from build123d import *

# Parameters (mm, degrees)
SKETCH_1_W          = 44.75
SKETCH_1_H          = 50
EXTRUDE_1_DEPTH     = 30
SHELL_1_T           = 5
FILLET_1_R          = 5
SKETCH_2_R          = 0.75
CUT_EXTRUDE_1_DEPTH = 70.264438928
SKETCH_3_R          = 5
CUT_EXTRUDE_2_DEPTH = 70.264438928
EXTRUDE_2_DEPTH     = 30
CUT_EXTRUDE_3_DEPTH = 20
SKETCH_7_R          = 2.1
CUT_EXTRUDE_4_DEPTH = 159.731347329
SKETCH_8_W          = 18
SKETCH_8_H          = 45
CUT_EXTRUDE_5_DEPTH = 10
SKETCH_9_W          = 18
SKETCH_9_H          = 45
CUT_EXTRUDE_6_DEPTH = 10
FILLET_2_R          = 3


with BuildPart() as part:
    # 草图1 → 凸台-拉伸1 (new body)
    with BuildSketch(Plane.XY):
        Rectangle(SKETCH_1_W, SKETCH_1_H)
    extrude(amount=EXTRUDE_1_DEPTH)

    # 抽壳1
    shell_1_openings = [part.faces().sort_by_distance(p)[0] for p in [
        (0, -25, 15),
        (0, 0, 0),
        (0, 0, 30),
    ]]
    offset(amount=SHELL_1_T, openings=shell_1_openings, kind=Kind.INTERSECTION)

    # 圆角1
    # the kernel refuses this fillet: 5 mm, written as the material it takes off along each edge
    with BuildSketch(Plane(origin=(-27.375, 30, -12.5), x_dir=(1, 0, 0), z_dir=(0, 0, 1)), Plane(origin=(-27.375, -25, 42.5), x_dir=(1, 0, 0), z_dir=(0, 0, -1)), Plane(origin=(27.375, -25, -12.5), x_dir=(-1, 0, 0), z_dir=(0, 0, 1)), Plane(origin=(27.375, 30, 42.5), x_dir=(-1, 0, 0), z_dir=(0, 0, -1))) as fillet_1_piece_1:
        with BuildLine():
            CenterArc((FILLET_1_R, -FILLET_1_R), FILLET_1_R, 90, 90)
            Line((0, -FILLET_1_R), (0, 0))
            Line((0, 0), (FILLET_1_R, 0))
        make_face()
    extrude(amount=55, mode=Mode.SUBTRACT)
    with BuildSketch(Plane(origin=(-27.375, -37.5, 30), x_dir=(1, 0, 0), z_dir=(0, 1, 0)), Plane(origin=(27.375, 42.5, 30), x_dir=(-1, 0, 0), z_dir=(0, -1, 0))) as fillet_1_piece_2:
        with BuildLine():
            CenterArc((FILLET_1_R, FILLET_1_R), FILLET_1_R, 180, 90)
            Line((0, FILLET_1_R), (0, 0))
            Line((0, 0), (FILLET_1_R, 0))
        make_face()
    extrude(amount=80, mode=Mode.SUBTRACT)
    with BuildSketch(Plane(origin=(-27.375, -37.5, 0), x_dir=(1, 0, 0), z_dir=(0, 1, 0)), Plane(origin=(27.375, 42.5, 0), x_dir=(-1, 0, 0), z_dir=(0, -1, 0))) as fillet_1_piece_3:
        with BuildLine():
            CenterArc((FILLET_1_R, -FILLET_1_R), FILLET_1_R, 90, 90)
            Line((0, -FILLET_1_R), (0, 0))
            Line((0, 0), (FILLET_1_R, 0))
        make_face()
    extrude(amount=80, mode=Mode.SUBTRACT)

    # 草图2 → 切除-拉伸1 (cut, through all)
    with BuildSketch(Plane.ZY.offset(27.375)):
        with Locations(Location((15, 7, 0), (0, 0, 270))):
            Circle(SKETCH_2_R)
        with Locations(Location((12, 7, 0), (0, 0, 270))):
            Circle(SKETCH_2_R)
        with Locations(Location((18, 7, 0), (0, 0, 270))):
            Circle(SKETCH_2_R)
        with Locations(Location((8, -3, 0), (0, 0, 90))):
            Circle(SKETCH_2_R)
        with Locations(Location((8, 0, 0), (0, 0, 90))):
            Circle(SKETCH_2_R)
        with Locations(Location((8, 3, 0), (0, 0, 90))):
            Circle(SKETCH_2_R)
        with Locations(Location((12, -7, 0), (0, 0, 90))):
            Circle(SKETCH_2_R)
        with Locations(Location((15, -7, 0), (0, 0, 90))):
            Circle(SKETCH_2_R)
        with Locations(Location((18, -7, 0), (0, 0, 90))):
            Circle(SKETCH_2_R)
        with Locations(Location((22, -3, 0), (0, 0, 270))):
            Circle(SKETCH_2_R)
        with Locations(Location((22, 0, 0), (0, 0, 270))):
            Circle(SKETCH_2_R)
        with Locations(Location((22, 3, 0), (0, 0, 270))):
            Circle(SKETCH_2_R)
    extrude(amount=-CUT_EXTRUDE_1_DEPTH, mode=Mode.SUBTRACT)

    # 草图3 → 切除-拉伸2 (cut, through all)
    with BuildSketch(Plane(origin=(27.375, 0, 0), x_dir=(0, 0, -1), z_dir=(1, 0, 0))):
        with Locations(Location((-15, 0, 0), (0, 0, 90))):
            Circle(SKETCH_3_R)
    extrude(amount=-CUT_EXTRUDE_2_DEPTH, mode=Mode.SUBTRACT)

    # 草图4 → 凸台-拉伸2 (add)
    with BuildSketch(Plane.XY.offset(30)):
        Polygon((0, 30), (-15, 30), (-15, 150), (15, 150), (15, 30), align=None)
    extrude(amount=-EXTRUDE_2_DEPTH)

    # 草图6 → 切除-拉伸3 (cut)
    with BuildSketch(Plane.XY.offset(30)):
        Polygon((-15, 99), (15, 99), (15, 141), (5, 141), (5, 150), (-15, 150), (-15, 141), align=None)
    extrude(amount=-CUT_EXTRUDE_3_DEPTH, mode=Mode.SUBTRACT)

    # 草图7 → 切除-拉伸4 (cut, through all)
    with BuildSketch(Plane(origin=(15, 0, 0), x_dir=(0, 0, -1), z_dir=(1, 0, 0))):
        with Locations((-24.925, 144.75)):
            Circle(SKETCH_7_R)
        with Locations((-15.075, 144.75)):
            Circle(SKETCH_7_R)
        with Locations(Location((-15.075, 95.25, 0), (0, 0, 180))):
            Circle(SKETCH_7_R)
        with Locations(Location((-24.925, 95.25, 0), (0, 0, 180))):
            Circle(SKETCH_7_R)
    extrude(amount=-CUT_EXTRUDE_4_DEPTH, mode=Mode.SUBTRACT)

    # 草图8 → 切除-拉伸5 (cut)
    with BuildSketch(Plane.XY.offset(30)):
        with Locations((0, 64.5)):
            Rectangle(SKETCH_8_W, SKETCH_8_H)
    extrude(amount=-CUT_EXTRUDE_5_DEPTH, mode=Mode.SUBTRACT)

    # 草图9 → 切除-拉伸6 (cut)
    with BuildSketch(Plane(origin=(0, 0, 0), x_dir=(-1, 0, 0), z_dir=(0, 0, -1))):
        with Locations((0, 65)):
            Rectangle(SKETCH_9_W, SKETCH_9_H)
    extrude(amount=-CUT_EXTRUDE_6_DEPTH, mode=Mode.SUBTRACT)

    # 圆角2
    fillet_2_edges = [part.edges().sort_by_distance(p)[0] for p in [
        (-15, 90, 0),
        (15, 90, 0),
        (15, 64.5, 30),
        (-15, 64.5, 30),
    ]]
    fillet(fillet_2_edges, radius=FILLET_2_R)


solid = part.part
Geometry check sheet. Reference: the model listing, model coordinates, mm. A direction names the side the tool comes from. Give positions to 0.01 mm unless a question says otherwise; leave off trailing zeros. Loops run counter-clockwise (first coordinate to the right, second up) from the corner with the lowest first, then second, coordinate; pieces in that order, holes last. Notation, with made-up numbers: (64.25, -27.5) -> (97.25, -27.5) arc R4 ccw to (97.25, -21.5) -> close; hole circle Ø4 at (36.5, 75). An arc over 180 degrees is marked (long way). Answer in a Markdown table with one row per item. Add a question column.
1) Cross-section at C-C on y = -10.5. Record the boundary of the cut face in (x, z) (3 decimals).
2) Cross-section at D-D on y = 103. Record the boundary of the cut face in (x, z), and give its area (3 significant figures).
3) Cross-section at B-B on x = 6.5. Record the boundary of the cut face in (y, z) (3 decimals), and give its area (3 significant figures).
4) Set-up check for faces 4 (the face through (5, 145, 20)), 5 (the face through (0, 87.5, 5)), 6 (the face through (14.1, 89.16, 0.86)), 7 (the face through (-22.375, -6, 15)): record each of +Z, -Z, +X, -X, +Y, -Y from which the full face is reachable in a straight line by a thin tool's end or side.
5) Gauge pin test, flat ends, axial feed: P1, Ø2, axis at y = 54.5, z = 8, coming from the +X side; P2, Ø7, axis at y = 145, z = 23, coming from the -X side; P3, Ø10, axis at x = -19.5, z = 17.5, coming from the +Y side. Record the tip position at first contact, or that the pin passes through.
6) Material ranges on probe 1 along Z at (x, y) = (8, 95); probe 2 along Y at (x, z) = (14, 27.5); probe 3 along Y at (x, z) = (-12, 25), recorded low to high. Write a range as from..to.
7) Draft check along Y on faces 1 (the face through (10.07, 146.83, 15.35)), 2 (the face through (-14.1, 62.92, 29.14)), 3 (the face through (25.871, 28.574, 15.21)). Enter one of: pulls with the +Y half, pulls with the -Y half, needs draft (parallel to the pull), parting line crosses it, or undercut.
8) Cross-section at A-A on y = 144.75. Record the boundary of the cut face in (x, z) (3 decimals).
Outcome:
| question | item | result |
|---|---|---|
| 1 | outline | (-27.375, 5) arc R5 ccw to (-22.375, 0) -> (-22.375, 30) arc R5 ccw to (-27.375, 25) -> close; (22.375, 0) arc R5 ccw to (27.375, 5) -> (27.375, 25) arc R5 ccw to (22.375, 30) -> close |
| 2 | outline | (-15, 3) arc R3 ccw to (-12, 0) -> (12, 0) arc R3 ccw to (15, 3) -> (15, 10) -> (-15, 10) -> close |
| 2 | area | 296 mm^2 |
| 3 | outline | (25, 0) -> (42.5, 0) -> (42.5, 10) -> (87.5, 10) -> (87.5, 0) -> (150, 0) -> (150, 30) -> (141, 30) -> (141, 10) -> (99, 10) -> (99, 30) -> (87, 30) -> (87, 20) -> (42, 20) -> (42, 30) -> (25, 30) -> close; hole circle Ø4.2 at (95.25, 15.075); hole circle Ø4.2 at (95.25, 24.925); hole circle Ø4.2 at (144.75, 15.075); hole circle Ø4.2 at (144.75, 24.925) |
| 3 | area | 1,950 mm^2 |
| 4 | face 4 | +Z, -X, +Y |
| 4 | face 5 | -Z |
| 4 | face 6 | -Z, +X, +Y |
| 4 | face 7 | +Z, -Z, -Y |
| 5 | P1 | stops at x = 15 |
| 5 | P2 | stops at x = 5 |
| 5 | P3 | stops at y = 99 |
| 6 | probe 1 | z = 0..12.99, 17.16..22.84, 27.01..30 |
| 6 | probe 2 | y = 25..99, 141..150 |
| 6 | probe 3 | y = 25..93.15, 97.35..99 |
| 7 | face 1 | undercut |
| 7 | face 2 | needs draft |
| 7 | face 3 | pulls with the +Y half |
| 8 | outline | (-15, 3) arc R3 ccw to (-12, 0) -> (12, 0) arc R3 ccw to (15, 3) -> (15, 12.975) -> (5, 12.975) -> (5, 10) -> (-15, 10) -> close; (5, 17.175) -> (15, 17.175) -> (15, 22.825) -> (5, 22.825) -> close; (5, 27.025) -> (15, 27.025) -> (15, 30) -> (5, 30) -> close |
